Could you check a few things on this model? Use its own coordinates, in mm. Face numbers are marked on the shaded views. A direction names the side the tool comes from. Give positions to 0.01 mm unless a question says otherwise; leave off trailing zeros. Order: outer loops, then holes, each group sorted by start corner. A loop starts at its lowest first (then second) coordinate and runs counter-clockwise, first axis right, second up. Notation, with made-up numbers: (23, -39) - (52, -39) arc R25 cw to (52, 0) - close; hole circle Ø2 at (24.5, 38.25). An arc over 180 degrees is marked (long way). One line per question, with ' | ' between items. Start each with the question number.
1. Which directions (+Z, -Z, +X, -X, +Y, -Y) give clear straight access to the entire face, cutting with the end or side of a thin tool? Please do the marked faces 1 and 2.
2. I need wall thicknesses on probe 1 along Y at (x, z) = (-1, 7); probe 2 along X at (y, z) = (11.5, 1); probe 3 along X at (y, z) = (34.5, 7). Which ranges of each line are inside material? Lowest first, please. Write a range as from..to.
3. Imagine slicing it at B-B (y = -63.5). Please give me the cut outline in (x, z).
4. Imagine slicing it at C-C (z = -0.5). Please give me the cut outline in (x, y).
5. Imagine slicing it at A-A (x = 0). Please give me the cut outline in (y, z).
6. For P1, Ø2, axis at x = 18.5, z = 14, coming from the +Y side; P2, Ø7, axis at y = 64, z = 2.5, coming from the -X side; P3, Ø8, axis at x = -27, y = 37, coming from the +Z side, each with a flat end and sliding along its axis, tell me the tip position at first contact or that it passes through.
7. Imagine slicing it at D-D (z = 16.5). Please give me the cut outline in (x, y), and give its area (3 significant figures).
8. If we mould it in two halves opening along Y, with no side actions, what happens to the marked faces 3, 4, 5 and 6? For each: released by +Y, released by -Y, zero draft, split by the parting line, or undercut.
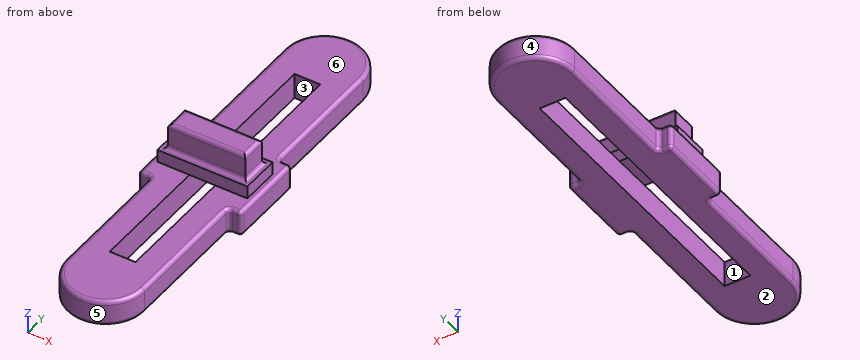
```python
from build123d import *

# Parameters (mm, degrees)
SKETCH1_W           = 20
SKETCH1_H           = 220
BOSS_EXTRUDE1_DEPTH = 10
SKETCH2_W           = 60
SKETCH2_H           = 20
BOSS_EXTRUDE2_DEPTH = 30
SKETCH3_W           = 69.73889917
SKETCH3_H           = 30
SKETCH3_W_2         = 60
SKETCH3_H_2         = 20
BOSS_EXTRUDE3_DEPTH = 10
FILLET2_R           = 3


with BuildPart() as part:
    # Sketch1 → Boss-Extrude1 (new, symmetric)
    with BuildSketch(Plane.XY):
        with BuildLine():
            Line((30, 130), (30, 30))
            Line((30, 30), (40, 30))
            Line((40, 30), (40, -30))
            Line((40, -30), (30, -30))
            Line((30, -30), (30, -130))
            ThreePointArc((30, -130), (0, -160), (-30, -130))
            Line((-30, -130), (-30, -30))
            Line((-30, -30), (-40, -30))
            Line((-40, -30), (-40, 30))
            Line((-40, 30), (-30, 30))
            Line((-30, 30), (-30, 130))
            ThreePointArc((-30, 130), (0, 160), (30, 130))
        make_face()
        Rectangle(SKETCH1_W, SKETCH1_H, mode=Mode.SUBTRACT)
    extrude(amount=BOSS_EXTRUDE1_DEPTH, both=True)

    # Sketch2 → Boss-Extrude2 (add)
    with BuildSketch(Plane.XY.offset(10)):
        Rectangle(SKETCH2_W, SKETCH2_H)
    extrude(amount=BOSS_EXTRUDE2_DEPTH)

    # Sketch3 → Boss-Extrude3 (add)
    with BuildSketch(Plane.XY.offset(10)):
        Rectangle(SKETCH3_W, SKETCH3_H)
        Rectangle(SKETCH3_W_2, SKETCH3_H_2, mode=Mode.SUBTRACT)
    extrude(amount=BOSS_EXTRUDE3_DEPTH)

    # Fillet2
    fillet2_edges = [part.edges().sort_by_distance(p)[0] for p in [
        (30, 80, -10),
        (35, 30, -10),
        (-35, 30, 10),
        (40, 0, -10),
        (35, -30, -10),
        (30, -80, -10),
        (0, -160, -10),
        (-30, -80, -10),
        (-35, -30, -10),
        (-40, 0, -10),
        (-35, 30, -10),
        (-30, 80, -10),
        (0, 160, -10),
        (-40, 0, 10),
        (30, 30, 0),
        (40, 30, 0),
        (-35, -30, 10),
        (40, -30, 0),
        (30, -30, 0),
        (-30, -30, 0),
        (-40, -30, 0),
        (-40, 30, 0),
        (-30, 30, 0),
        (-30, -80, 10),
        (0, -160, 10),
        (30, -80, 10),
        (35, -30, 10),
        (40, 0, 10),
        (35, 30, 10),
        (30, 80, 10),
        (0, 160, 10),
        (30, 0, 40),
        (0, 10, 40),
        (-30, 0, 40),
        (0, -10, 40),
        (30, 0, 20),
        (0, 10, 20),
        (-30, 0, 20),
        (0, -10, 20),
        (-30, 80, 10),
    ]]
    fillet(fillet2_edges, radius=FILLET2_R)


solid = part.part
```
Results found:
1) face 1: +Z, -Z | face 2: -Z, +X, -X, +Y, -Y
2) probe 1: y = -159.98..-110, 110..159.98 | probe 2: x = -40..-10, 10..40 | probe 3: x = -30..-10, 10..30
3) outline: (-30, -7) arc R3 ccw to (-27, -10) - (-10, -10) - (-10, 10) - (-27, 10) arc R3 ccw to (-30, 7) - close; (10, -10) - (27, -10) arc R3 ccw to (30, -7) - (30, 7) arc R3 ccw to (27, 10) - (10, 10) - close
4) outline: (-40, -27) arc R3 ccw to (-37, -30) - (-33, -30) arc R3 cw to (-30, -33) - (-30, -130) arc R30 ccw to (30, -130) - (30, -33) arc R3 cw to (33, -30) - (37, -30) arc R3 ccw to (40, -27) - (40, 27) arc R3 ccw to (37, 30) - (33, 30) arc R3 cw to (30, 33) - (30, 130) arc R30 ccw to (-30, 130) - (-30, 33) arc R3 cw to (-33, 30) - (-37, 30) arc R3 ccw to (-40, 27) - close; hole (-10, -110) - (10, -110) - (10, 110) - (-10, 110) - close
5) outline: (-160, -7) arc R3 ccw to (-157, -10) - (-110, -10) - (-110, 10) - (-157, 10) arc R3 ccw to (-160, 7) - close; (-15, 10) - (15, 10) - (15, 20) - (13, 20) arc R3 cw to (10, 23) - (10, 37) arc R3 ccw to (7, 40) - (-7, 40) arc R3 ccw to (-10, 37) - (-10, 23) arc R3 cw to (-13, 20) - (-15, 20) - close; (110, -10) - (157, -10) arc R3 ccw to (160, -7) - (160, 7) arc R3 ccw to (157, 10) - (110, 10) - close
6) P1: stops at y = 15 | P2: stops at x = -30 | P3: stops at z = 10
7) outline: (-34.87, -15) - (34.87, -15) - (34.87, 15) - (-34.87, 15) - close | area: 2,090 mm2
8) face 3: undercut | face 4: released by +Y | face 5: released by -Y | face 6: zero draft
